Could you check a few things on this model? Use its own coordinates, in mm. A direction names the side the tool comes from. Round coordinates to 2 decimals unless told otherwise and drop trailing zeros. Loops run counter-clockwise (first coordinate to the right, second up) from the corner with the lowest first, then second, coordinate; pieces in that order, holes last. Notation, with made-up numbers: (71.5, -0.75) -> (80.5, -0.75) arc R33 ccw to (80.5, 33.25) -> close; hole circle Ø11 at (28.5, 8.5). An arc over 180 degrees is marked (long way). One line per item, written item: value.
```python
from build123d import *

# Parameters (mm, degrees)
F0_R      = 15.24
F0_R_2    = 12.7
F1_DEPTH  = 12.7
F0_R_3    = 19.05
F2_DEPTH  = 2.54
F5_R      = 15.24
F4_R      = 8.89
F7_R      = 8.89
F7_R_2    = 6.35
F8_DEPTH  = 2.54
F9_R      = 12.7
F9_R_2    = 6.35
F10_DEPTH = 2.54
F11_DEPTH = 41.402


# Not quite as in the source:
# - a fillet or chamfer that OpenCascade refuses, or shapes differently, is made with other operations: its cross-section is extruded or revolved along the edge and cut away or added


with BuildPart() as f1:
    # F0 (on Front) → F1 (new body)
    with BuildSketch(Plane.XZ):
        Circle(F0_R)
        Circle(F0_R_2, mode=Mode.SUBTRACT)
    extrude(amount=F1_DEPTH)

    # F0 (on Front) → F2 (join)
    with BuildSketch(Plane.XZ):
        Circle(F0_R_3)
        Circle(F0_R, mode=Mode.SUBTRACT)
    extrude(amount=F2_DEPTH)

    # F5 (on face) → F6 section 0
    with BuildSketch(Plane.XZ.offset(12.7)):
        Circle(F5_R)
    # F4 (on offset) → F6 section 1
    with BuildSketch(Plane.XZ.offset(50.8)):
        Circle(F4_R)
    loft()

    # F7 (on face) → F8 (join)
    with BuildSketch(Plane.XZ.offset(50.8)):
        Circle(F7_R)
        Circle(F7_R_2, mode=Mode.SUBTRACT)
    extrude(amount=F8_DEPTH)

    # F9 (on face) → F10 (join)
    with BuildSketch(Plane.XZ.offset(53.34)):
        Circle(F9_R)
        Circle(F9_R_2, mode=Mode.SUBTRACT)
    extrude(amount=F10_DEPTH)

    # F11 (cut): a face of the model
    f11_faces = [f1.faces().sort_by_distance(p)[0] for p in [
        (0, -50.8, 0),
    ]]
    extrude(f11_faces, amount=-F11_DEPTH, mode=Mode.SUBTRACT)

    # F12: fillet of radius 25.4 on 1 edges, made by hand

    # F12_s1 → F12_t2 (revolve, cut)
    with BuildSketch(Plane.XY):
        with BuildLine():
            ThreePointArc((12.7, -12.7), (7.990475594, -20.5202647042), (6.35, -29.5005208253))
            Line((6.35, -29.5005208253), (5.842, -29.5005208253))
            Line((5.842, -29.5005208253), (5.842, -12.7))
            Line((5.842, -12.7), (6.35, -12.192))
            ThreePointArc((6.35, -12.192), (9.525, -12.192), (12.319, -12.3639895835))
            Line((12.319, -12.3639895835), (12.7, -12.7))
        make_face()
    revolve(axis=Axis((0, -12.7, 0), (0, -1, 0)), mode=Mode.SUBTRACT)


solid = f1.part
```
(1) Please list where these lines run through material, in increasing order: L1, parallel to Z at x = 0, y = -52; L2, parallel to Z at x = 0, y = -54; L3, parallel to X at y = -30, z = -1.5.
Results below:
L1: z = -8.89 to -6.35, 6.35 to 8.89
L2: z = -12.7 to -6.35, 6.35 to 12.7
L3: x = -12.27 to -6.17, 6.17 to 12.27
(2) For pin 1 Ø2 at (x, z) = (0.5, 13) entering from +Y; pin 2 Ø7.5 at (x, z) = (-4, -4) entering from +Y; pin 3 Ø10 at (x, z) = (0, 0) entering from -Y; pin 4 Ø1.5 at (x, z) = (-4.5, 9.5) entering from +Y, each with a flat end and sliding along its axis, tell me the tip position at first contact or that it passes through.
Results below:
pin 1: stops at y = 0
pin 2: stops at y = -17.42
pin 3: passes through
pin 4: stops at y = -14.49
(3) We'd pull the mould along Y, two halves only. Please class faces 1 (the face through (-3.3, -7.55, -14.88)), 2 (the face through (3, -55.88, 6)), 3 (the face through (-9, -53.34, -3)): +Y half, -Y half, draft (parallel to the pull), parting line (faces both ways), or undercut.
Results below:
face 1: draft
face 2: -Y half
face 3: undercut
(4) On a 3-axis mill with a long thin cutter (end or side, diameter ignored), from which of +Z, -Z, +X, -X, +Y, -Y can I reach the whole of each face in a straight line? I mean faces 4 (the face through (-2.75, -6.26, -12.4)), 5 (the face through (-9, -2.54, 13)), 6 (the face through (-1.93, -52.05, -8.68)). Say none if no direction works.
Results below:
face 4: +Y
face 5: -Y
face 6: none
(5) Imagine slicing it at D-D on x = 16.5. Write out the boundary of the cut face in (y, z).
Results below:
outline: (-2.54, -9.52) -> (0, -9.52) -> (0, 9.52) -> (-2.54, 9.52) -> close
(6) Imagine slicing it at B-B on y = -34. Write out the boundary of the cut face in (x, z).
Results below:
outline: circle Ø23.38 at (0, 0); hole circle Ø12.7 at (0, 0)
(7) Imagine slicing it at A-A on x = 0. Write out the boundary of the cut face in (y, z), then the cut area to 3 significant figures.
Results below:
outline: (-55.88, -12.7) -> (-53.34, -12.7) -> (-53.34, -8.89) -> (-50.8, -8.89) -> (-12.7, -15.24) -> (-2.54, -15.24) -> (-2.54, -19.05) -> (0, -19.05) -> (0, -12.7) -> (-12.7, -12.7) arc R25.4 ccw to (-29.5, -6.35) -> (-55.88, -6.35) -> close; (-55.88, 6.35) -> (-29.5, 6.35) arc R25.4 ccw to (-12.7, 12.7) -> (0, 12.7) -> (0, 19.05) -> (-2.54, 19.05) -> (-2.54, 15.24) -> (-12.7, 15.24) -> (-50.8, 8.89) -> (-53.34, 8.89) -> (-53.34, 12.7) -> (-55.88, 12.7) -> close
area: 497 mm²
(8) Imagine slicing it at C-C on y = -51.5. Write out the boundary of the cut face in (x, z).
Results below:
outline: circle Ø17.78 at (0, 0); hole circle Ø12.7 at (0, 0)
